from build123d import *

# Parameters (mm, degrees)
BOSS_EXTRUDE1_DEPTH = 3


with BuildPart() as part:
    # Sketch1 → Boss-Extrude1 (new body)
    with BuildSketch(Plane(origin=(0, 0, 0), x_dir=(1, 0, 0), z_dir=(0, 1, 0))):
        with BuildLine():
            Line((-5, 30), (-5, 5.590169944))
            ThreePointArc((-5, 5.590169944), (0, 7.5), (5, 5.590169944))
            Line((5, 5.590169944), (5, 30))
            ThreePointArc((5, 30), (0, 35), (-5, 30))
        make_face()
        with BuildLine():
            ThreePointArc((-1.25, 30), (0, 31.25), (1.25, 30))
            Line((1.25, 30), (1.25, 10))
            ThreePointArc((1.25, 10), (0, 8.75), (-1.25, 10))
            Line((-1.25, 10), (-1.25, 30))
        make_face(mode=Mode.SUBTRACT)
        with BuildLine():
            ThreePointArc((5, 0), (0, -5), (-5, 0))
            Line((-5, 0), (-5, 5.590169944))
            ThreePointArc((-5, 5.590169944), (-3.061862178, -6.846531969), (7.5, 0))
            ThreePointArc((7.5, 0), (6.846531969, 3.061862178), (5, 5.590169944))
            Line((5, 5.590169944), (5, 0))
        make_face()
        with BuildLine():
            Line((-5, 5.590169944), (-5, 0))
            ThreePointArc((-5, 0), (0, -5), (5, 0))
            Line((5, 0), (5, 5.590169944))
            ThreePointArc((5, 5.590169944), (0, 7.5), (-5, 5.590169944))
        make_face()
    extrude(amount=BOSS_EXTRUDE1_DEPTH)


solid = part.part
The model under review builds one solid part; all positions refer to its coordinate system, in mm. A direction names the side the tool comes from. Coordinates: 2 decimals unless noted, no trailing zeros. Loops run counter-clockwise (first coordinate to the right, second up) from the corner with the lowest first, then second, coordinate; pieces in that order, holes last.
(1) Wall thickness on L1, parallel to Z at x = 0, y = 1.4; L2, parallel to X at y = 2.65, z = -13.5; L3, parallel to Z at x = -0.5, y = 0.45: over which ranges is each line inside the solid? List them lowest first.
Determined:
L1: z = -35 to -31.25, -8.75 to 7.5
L2: x = -5 to -1.25, 1.25 to 5
L3: z = -34.97 to -31.15, -8.85 to 7.48
(2) Insertion check: P1, Ø1.5, axis at y = 1, z = -12.5, coming from the +X side; P2, Ø1.5, axis at y = 1, z = -12, coming from the -X side; P3, Ø1.5, axis at x = -3, y = 2, coming from the +Z side. Each pin has a flat end and moves straight along its axis. Give the tip position at first contact, or say it passes through.
Determined:
P1: stops at x = 5
P2: stops at x = -5
P3: stops at z = 7.15
(3) Consider section B-B, the plane y = 2.45. Give the boundary of the cut face in (x, z).
Determined:
outline: (-5, -30) arc R5 ccw to (5, -30) - (5, -5.59) arc R7.5 ccw (long way) to (-5, -5.59) - close; hole (-1.25, -30) arc R1.25 ccw to (1.25, -30) - (1.25, -10) arc R1.25 ccw to (-1.25, -10) - close
(4) Consider section A-A, the plane z = -24.5. Give the boundary of the cut face in (x, y).
Determined:
outline: (-5, 0) - (-1.25, 0) - (-1.25, 3) - (-5, 3) - close; (1.25, 0) - (5, 0) - (5, 3) - (1.25, 3) - close
(5) Consider section C-C, the plane x = 0.25. Give the boundary of the cut face in (y, z), plus the area to 3 significant figures.
Determined:
outline: (0, -34.99) - (3, -34.99) - (3, -31.22) - (0, -31.22) - close; (0, -8.78) - (3, -8.78) - (3, 7.5) - (0, 7.5) - close
area: 60.1 mm2
(6) Draft analysis for pull direction X (two halves, no side actions). For faces 1 (the cylindrical face through (0, 1, -35)), 2 (the cylindrical face through (-0.03, 1.48, -31.25)), 3 (the flat face through (-5, 1, -18)), state which applies: +X half, -X half, draft (parallel to the pull), parting line (faces both ways), or undercut.
Determined:
face 1: parting line
face 2: undercut
face 3: -X half
(7) Tool access review of faces 4 (the flat face through (5, 1, -18)), 5 (the flat face through (1.25, 1, -20)), 6 (the flat face through (2, 0, -14)): name each direction out of +Z, -Z, +X, -X, +Y, -Y from which nothing blocks a thin tool from reaching the whole face with its end or side.
Determined:
face 4: -Z, +X, +Y, -Y
face 5: +Y, -Y
face 6: +Z, -Z, +X, -X, -Y
(8) Consider section D-D, the plane x = -6.25. Give the boundary of the cut face in (y, z).
Determined:
outline: (0, -4.15) - (3, -4.15) - (3, 4.15) - (0, 4.15) - close
